from build123d import *

# Parameters (mm, degrees)
F0_W     = 30
F0_H     = 14
F0_R     = 2
F1_DEPTH = 2
F4_DEPTH = 2.5
F6_SIZE2 = 3.2708526185
F6_SIZE  = 1
F8_R     = 2.15
F9_DEPTH = 14.701


with BuildPart() as f1:
    # F0 (on Right) → F1 (new body)
    with BuildSketch(Plane.YZ):
        Rectangle(F0_W, F0_H)
        with Locations((-10, 0)):
            Circle(F0_R, mode=Mode.SUBTRACT)
        with Locations((10, 0)):
            Circle(F0_R, mode=Mode.SUBTRACT)
    extrude(amount=F1_DEPTH)

    # F3 (on offset) → F4 (join)
    with BuildSketch(Plane.XY.offset(7)):
        with BuildLine():
            ThreePointArc((4.0091983974, -15.0103159249), (17.5963547051, 0.0841872352), (3.8013714597, 14.9889944946))
            Line((3.8013714597, 14.9889944946), (0, 14.9889944946))
            Line((0, 14.9889944946), (0, -14.9888552843))
            Line((0, -14.9888552843), (4.0091983974, -15.0103159249))
        make_face()
    extrude(amount=-F4_DEPTH)

    # F5: F1 across plane


with BuildPart() as f1_1:
    add(f1.part)
    add(f1.part.mirror(Plane.XY))

    # F6
    f6_edges = [f1_1.edges().sort_by_distance(p)[0] for p in [
        (2, -0.005283, 4.5),
        (2, -0.005283, -4.5),
    ]]
    f6_side = f1_1.faces().sort_by_distance((2, 0.003234, 0))[0]
    chamfer(f6_edges, length=F6_SIZE, length2=F6_SIZE2, reference=f6_side)

    # F8 (on offset) → F9 (cut, through all)
    with BuildSketch(Plane.XY.offset(7.7)):
        with Locations((11, 0)):
            Circle(F8_R)
    extrude(amount=-F9_DEPTH, mode=Mode.SUBTRACT)


solid = f1_1.part
Design review of the part built by this model. Coordinates are the model's own, in mm. Round coordinates to 2 decimals unless told otherwise and drop trailing zeros. Order: outer loops, then holes, each group sorted by start corner. A loop starts at its lowest first (then second) coordinate and runs counter-clockwise, first axis right, second up. Notation, with made-up numbers: M 14.25,5.25 L 19.25,5.25 A29 ccw 19.25,32.25 Z; hole C -34,89.25 d8. An arc over 180 degrees is marked long. Answer as CSV lines item,"result". Start each with the question number.
1) Add section D-D (y = 0). Give the boundary of the cut face in (x, z), then the cut area to 3 significant figures.
2) Add section A-A (y = 10). Give the boundary of the cut face in (x, z).
3) The part is to be moulded in two halves that separate along Z. For faces 1 (the face through (1, -11.6, -1.2)), 2 (the face through (7, 0, 7)), 3 (the face through (13.05, 0.65, 5.77)), say which applies: +Z half, -Z half, draft (parallel to the pull), parting line (faces both ways), or undercut.
4) For pin 1 Ø1 at (x, z) = (0.5, -2) entering from -Y; pin 2 Ø3.5 at (y, z) = (10, 0) entering from +X; pin 3 Ø8 at (x, z) = (7.5, 1.5) entering from +Y; pin 4 Ø1.4 at (x, z) = (3, 5.5) entering from +Y, all flat-tipped, find the tip position at first contact; note any pin that passes through.
5) Wall thickness on line 1 along Z through (x, y) = (11.5, 8); line 2 along X through (y, z) = (1, 2.25); line 3 along Y through (x, z) = (11, 6.15): over which ranges is each line inside the solid? List them lowest first. Write a range as [from, to].
6) Add section B-B (x = 5.75). Give the boundary of the cut face in (y, z), then the cut area to 3 significant figures.
Resolved:
1,outline,"M 0,-7 L 8.85,-7 L 8.85,-4.5 L 5.27,-4.5 L 2,-3.5 L 2,3.5 L 5.27,4.5 L 8.85,4.5 L 8.85,7 L 0,7 Z; M 13.15,-7 L 17.6,-7 L 17.6,-4.5 L 13.15,-4.5 Z; M 13.15,4.5 L 17.6,4.5 L 17.6,7 L 13.15,7 Z"
1,area,"87.8 mm^2"
2,outline,"M 0,-7 L 13.78,-7 L 13.78,-4.5 L 5.27,-4.5 L 2,-3.5 L 2,-2 L 0,-2 Z; M 0,2 L 2,2 L 2,3.5 L 5.27,4.5 L 13.78,4.5 L 13.78,7 L 0,7 Z"
3,face 1,"undercut"
3,face 2,"+Z half"
3,face 3,"draft"
4,pin 1,"y = -15"
4,pin 2,"through"
4,pin 3,"y = 14.89"
4,pin 4,"y = 14.99"
5,line 1,"[-7, -4.5], [4.5, 7]"
5,line 2,"[0, 2]"
5,line 3,"[-12.48, -2.15], [2.15, 12.44]"
6,outline,"M -14.74,-7 L 14.7,-7 L 14.7,-4.5 L -14.74,-4.5 Z; M -14.74,4.5 L 14.7,4.5 L 14.7,7 L -14.74,7 Z"
6,area,"147 mm^2"
